Build history of the part. All positions in model axes, mm. Face numbers are marked on the shaded views. Round coordinates to 2 decimals unless told otherwise and drop trailing zeros. Loops run counter-clockwise (first coordinate to the right, second up) from the corner with the lowest first, then second, coordinate; pieces in that order, holes last. Notation, with made-up numbers: (23, -36) -> (79, -36) arc R7 cw to (79, -26) -> close; hole circle Ø4 at (-8, -14.75). An arc over 180 degrees is marked (long way). Put each result on its own line as item: value. Start each with the question number.
Item 1: Cut at B-B, the plane z = 1.25. List the corners of the cut face in (x, y), plus the area to 3 significant figures.
Item 2: Cut at A-A, the plane x = 0. List the corners of the cut face in (y, z).
Item 3: Drill centre lines: probe 1 along Y at (x, z) = (0, 2.75); probe 2 along Y at (x, z) = (0.5, 6.75); probe 3 along X at (y, z) = (9.5, 0.5). Where is each one in solid material? Low to high. Write a range as [from, to].
Item 4: Cut at C-C, the plane y = -8.6. List the corners of the cut face in (x, z).
Item 5: Pull direction X, two halves, no side cores. Call the marked faces 1, 2 and 3: +X half, -X half, draft (parallel to the pull), parting line (faces both ways), or undercut.
Item 6: Cut at D-D, the plane y = 0. List the corners of the cut face in (x, z).
Item 7: Flat gauge pins, fed straight in: pin 1 Ø2.5 at (x, y) = (14.9, -8.6) entering from +Z; pin 2 Ø4 at (x, y) = (-14.9, -8.6) entering from -Z; pin 3 Ø1.5 at (y, z) = (3.5, 4.5) entering from -X; pin 4 Ø4 at (y, z) = (19.5, 4.5) entering from -X. Where does each tip first touch, or does it go through?
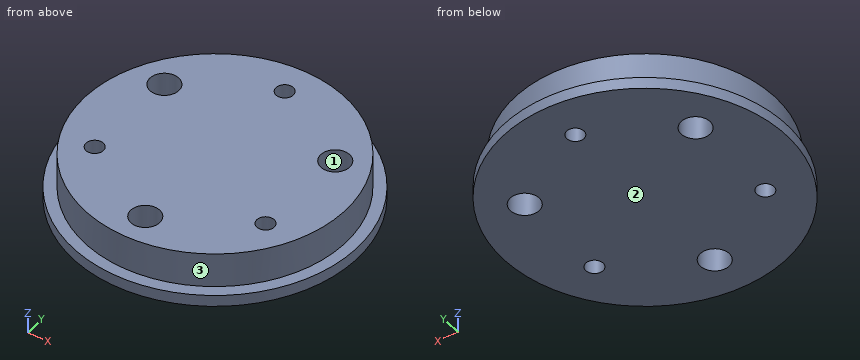
```python
from build123d import *

# Parameters (mm, degrees)
SKETCH1_R           = 24.5
SKETCH1_R_2         = 22.5
BOSS_EXTRUDE1_DEPTH = 2
SKETCH1_3_R         = 22.5
SKETCH1_3_R_2       = 2.5
SKETCH1_3_R_3       = 1.5
BOSS_EXTRUDE2_DEPTH = 8


with BuildPart() as part:
    # Sketch1 → Boss-Extrude1 (new body)
    with BuildSketch(Plane.XY):
        Circle(SKETCH1_R)
        Circle(SKETCH1_R_2, mode=Mode.SUBTRACT)
    extrude(amount=BOSS_EXTRUDE1_DEPTH)

    # Sketch1<3> → Boss-Extrude2 (add)
    with BuildSketch(Plane.XY):
        Circle(SKETCH1_3_R)
        with Locations((14.895636945, 8.6)):
            Circle(SKETCH1_3_R_2, mode=Mode.SUBTRACT)
        with Locations((-14.895636945, 8.6)):
            Circle(SKETCH1_3_R_2, mode=Mode.SUBTRACT)
        with Locations((0, -17.2)):
            Circle(SKETCH1_3_R_2, mode=Mode.SUBTRACT)
        with Locations((-14.895636945, -8.6)):
            Circle(SKETCH1_3_R_3, mode=Mode.SUBTRACT)
        with Locations((14.895636945, -8.6)):
            Circle(SKETCH1_3_R_3, mode=Mode.SUBTRACT)
        with Locations((0, 17.2)):
            Circle(SKETCH1_3_R_3, mode=Mode.SUBTRACT)
    extrude(amount=BOSS_EXTRUDE2_DEPTH)


solid = part.part
```
Reply:
1. outline: circle Ø49 at (0, 0); hole circle Ø5 at (-14.9, 8.6); hole circle Ø3 at (-14.9, -8.6); hole circle Ø5 at (0, -17.2); hole circle Ø3 at (0, 17.2); hole circle Ø5 at (14.9, 8.6); hole circle Ø3 at (14.9, -8.6)
1. area: 1,810 mm^2
2. outline: (-24.5, 0) -> (-19.7, 0) -> (-19.7, 8) -> (-22.5, 8) -> (-22.5, 2) -> (-24.5, 2) -> close; (-14.7, 0) -> (15.7, 0) -> (15.7, 8) -> (-14.7, 8) -> close; (18.7, 0) -> (24.5, 0) -> (24.5, 2) -> (22.5, 2) -> (22.5, 8) -> (18.7, 8) -> close
3. probe 1: y = [-22.5, -19.7], [-14.7, 15.7], [18.7, 22.5]
3. probe 2: y = [-22.49, -19.65], [-14.75, 15.79], [18.61, 22.49]
3. probe 3: x = [-22.58, -17.23], [-12.56, 12.56], [17.23, 22.58]
4. outline: (-22.94, 0) -> (-16.4, 0) -> (-16.4, 8) -> (-20.79, 8) -> (-20.79, 2) -> (-22.94, 2) -> close; (-13.4, 0) -> (13.4, 0) -> (13.4, 8) -> (-13.4, 8) -> close; (16.4, 0) -> (22.94, 0) -> (22.94, 2) -> (20.79, 2) -> (20.79, 8) -> (16.4, 8) -> close
5. face 1: undercut
5. face 2: draft
5. face 3: parting line
6. outline: (-24.5, 0) -> (24.5, 0) -> (24.5, 2) -> (22.5, 2) -> (22.5, 8) -> (-22.5, 8) -> (-22.5, 2) -> (-24.5, 2) -> close
7. pin 1: passes through
7. pin 2: stops at z = 0
7. pin 3: stops at x = -22.33
7. pin 4: stops at x = -14.14
